Print and shaded views of the part. All mm, measured from the part's lowest x, y and z. A direction names the side the tool comes from. Coordinates: 2 decimals unless noted, no trailing zeros. Loops run counter-clockwise (first coordinate to the right, second up) from the corner with the lowest first, then second, coordinate; pieces in that order, holes last. Notation, with made-up numbers: M 46,89 L 81,89 A20 ccw 81,94 Z; hole C 33,-2.75 d7. An arc over 180 degrees is marked long. Answer as CSV lines item,"result". Start each with the question number.
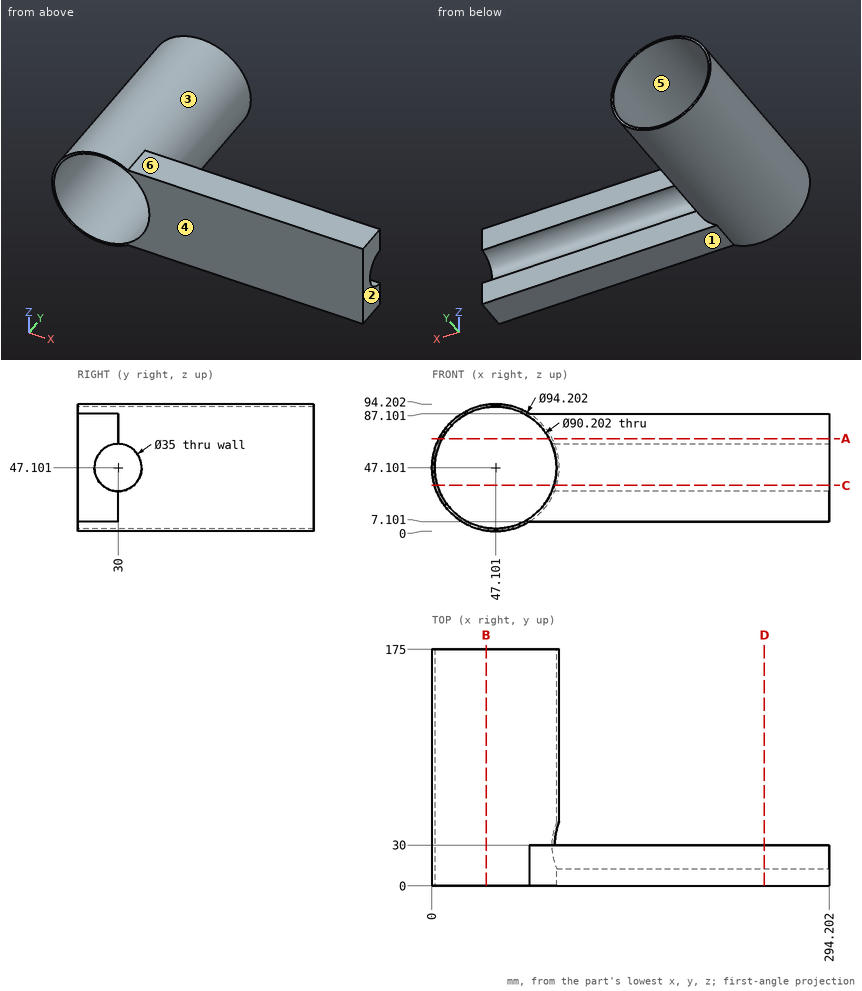
Q1. Slice it at D-D, the plane x = 246. Write the cut outline in (y, z), and give its area (3 significant figures).
Q2. Slice it at B-B, the plane x = 40. Write the cut outline in (y, z).
Q3. Two-plate mould, pull along Z, no slides. Class the marked faces 4, 5 and 6: +Z half, -Z half, draft (parallel to the pull), parting line (faces both ways), or undercut.
Q4. Slice it at A-A, the plane z = 68.5. Write the cut outline in (x, y).
Q5. Tool access for the marked faces 1, 2 and 3: list every direction of +Z, -Z, +X, -X, +Y, -Y with a clear straight run to the whole face (end or side of a thin tool).
Q6. Flat gauge pins, fed straight in: P1, Ø12, axis at x = 40, y = 32, coming from the -Z side; P2, Ø24, axis at x = 213, y = 11.5, coming from the -Z side; P3, Ø3, axis at x = 51, y = 78.5, coming from the +Z side. Where does each tip first touch, or does it go through?
Q7. Slice it at C-C, the plane z = 34. Write the cut outline in (x, y).
Q8. Wall check: L1, parallel to Y at x = 94.5, z = 74.5; L2, parallel to X at y = 78, z = 24; L3, parallel to X at y = 118, z = 80. Give the ranges that are in metal, low to high.
Solved:
1,outline,"M 0,7.1 L 30,7.1 L 30,29.6 A17.5 cw 30,64.6 L 30,87.1 L 0,87.1 Z"
1,area,"1,920 mm2"
2,outline,"M 0,0.54 L 175,0.54 L 175,2.56 L 0,2.56 Z; M 0,91.64 L 175,91.64 L 175,93.66 L 0,93.66 Z"
3,face 4,"draft"
3,face 5,"undercut"
3,face 6,"+Z half"
4,outline,"M 5.14,0 L 7.4,0 L 7.4,175 L 5.14,175 Z; M 86.8,0 L 294.2,0 L 294.2,30 L 89.06,30 L 89.06,175 L 86.8,175 Z"
5,face 1,"-Z, +X, +Y, -Y"
5,face 2,"+Z, -Z, +X, +Y, -Y"
5,face 3,"+Y"
6,P1,"stops at z = 0.01"
6,P2,"stops at z = 7.1"
6,P3,"stops at z = 94.14"
7,outline,"M 1.86,0 L 3.94,0 L 3.94,175 L 1.86,175 Z; M 90.26,0 L 294.2,0 L 294.2,18.4 L 90.26,18.4 Z; M 90.26,41.6 L 92.34,41.6 L 92.34,175 L 90.26,175 Z"
8,L1,"y = 0 to 30"
8,L2,"x = 6.05 to 8.37, 85.84 to 88.15"
8,L3,"x = 13.39 to 16.25, 77.95 to 80.81"
